Geometry check sheet. Reference: drawing and pictorial views, mm from the part's lowest x, y, z. Give positions to 0.01 mm unless a question says otherwise; leave off trailing zeros. Write each loop counter-clockwise with the first axis right and the second up, starting at its lowest first coordinate (ties: lowest second). Pieces come first, ordered by that corner, then holes. Notation, with made-up numbers: M 33.5,44.25 L 42.5,44.25 A28 cw 42.5,64.25 Z; hole C 15.5,36.25 d6. An arc over 180 degrees is marked long. Write item = value, one per line. Start each with the question number.
1) Cross-section at C-C, the plane z = 4.5. Record the cut outline in (x, y).
2) Scan lines: line 1 along Y through (x, z) = (165, 2.75); line 2 along X through (y, z) = (16.5, 7.25); line 3 along Y through (x, z) = (15, 5.75). Record each from-to range of solid material in increasing order. Write a range as [from, to].
3) Cross-section at A-A, the plane y = 15. Record the cut outline in (x, z), plus the area to 3 significant figures.
4) Cross-section at D-D, the plane x = 15. Record the cut outline in (y, z).
5) Cross-section at B-B, the plane x = 165. Record the cut outline in (y, z), plus the area to 3 significant figures.
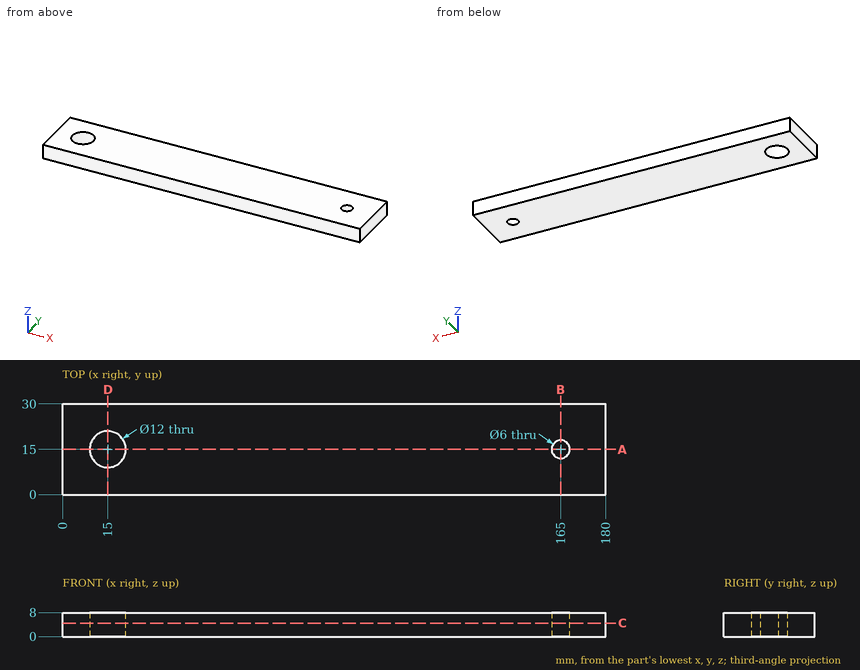
Reply:
q1.outline = M 0,0 L 180,0 L 180,30 L 0,30 Z; hole C 15,15 d12; hole C 165,15 d6
q2.line_1 = [0, 12], [18, 30]
q2.line_2 = [0, 9.19], [20.81, 162.4], [167.6, 180]
q2.line_3 = [0, 9], [21, 30]
q3.outline = M 0,0 L 9,0 L 9,8 L 0,8 Z; M 21,0 L 162,0 L 162,8 L 21,8 Z; M 168,0 L 180,0 L 180,8 L 168,8 Z
q3.area = 1,300 mm2
q4.outline = M 0,0 L 9,0 L 9,8 L 0,8 Z; M 21,0 L 30,0 L 30,8 L 21,8 Z
q5.outline = M 0,0 L 12,0 L 12,8 L 0,8 Z; M 18,0 L 30,0 L 30,8 L 18,8 Z
q5.area = 192 mm2
